Autodesk Inventor part; units mm, degrees
ref_plane "YZ Plane" through (0, 0, 0) normal (1, 0, 0) x (0, 1, 0)
ref_plane "XZ Plane" through (0, 0, 0) normal (0, 1, 0) x (-1, 0, 0)
ref_plane "XY Plane" through (0, 0, 0) normal (0, 0, 1) x (1, 0, 0)
sketch "Sketch1" plane through (0, 0, 0) normal (1, 0, 0) x (0, 1, 0)
  line L0 (44.45, 19.05) -> (-44.45, 19.05)
  line L1 (-44.45, 19.05) -> (-44.45, -19.05)
  line L2 (-44.45, -19.05) -> (44.45, -19.05)
  line L3 (44.45, -19.05) -> (44.45, 19.05)
  line L4 (44.45, 19.05) -> (-44.45, -19.05) construction
  line L5 (-44.45, 19.05) -> (44.45, -19.05) construction
  point P0 (0, 0)
  dimension "d0" = 88.9
  dimension "d1" = 38.1
extrude "Extrusion1" add sketch "Sketch1" along normal mid plane 410
sketch "Sketch2" plane through (-205, -44.45, 19.05) normal (0, 0, 1) x (1, 0, 0)
  line L0 (0, 88.9) -> (0, 0)
  line L1 (0, 67.1803) -> (192.497, 67.1803)
  line L2 (0, 88.9) -> (410, 88.9)
  line L3 (192.497, 88.9) -> (192.497, 67.1803)
  line L4 (192.497, 67.1803) -> (217.497, 67.1803)
  line L5 (217.497, 67.1803) -> (217.497, 88.9)
  point P0 (205, 44.45)
  dimension "d14" = 192.497
  dimension "d15" = 25
extrude "Extrusion2" cut sketch "Sketch2" against normal blind 166.2125 contours L2 L5 L4 L3
properties part number "CNC_1.1v_X_1(faceplate)"
Work out the finished part from the listing and answer in its coordinate system (mm). A direction names the side the tool comes from. Give positions to 0.01 mm unless a question says otherwise; leave off trailing zeros. Loops run counter-clockwise (first coordinate to the right, second up) from the corner with the lowest first, then second, coordinate; pieces in that order, holes last. Notation, with made-up numbers: (-34, -3) - (23, -3) arc R23 ccw to (23, 27) - close; hole circle Ø7 at (71.5, 17.5). An arc over 180 degrees is marked (long way). Answer in a Markdown table with one row per item.
(1) For a pull along X with two mould halves and no side action, classify faces 3 (the face through (205, -1, 0)), 4 (the face through (0, 22.73, 0)), 5 (the face through (-3, -1, -19.05)) as pulls with the +X half, pulls with the -X half, needs draft (parallel to the pull), parting line crosses it, or undercut.
Results list:
| item | result |
|---|---|
| face 3 | pulls with the +X half |
| face 4 | undercut |
| face 5 | needs draft |
(2) Section A-A (y = 36.5) is taken. Give the vertices of the cut face in (x, z).
Results list:
| item | result |
|---|---|
| outline | (-205, -19.05) - (-12.5, -19.05) - (-12.5, 19.05) - (-205, 19.05) - close; (12.5, -19.05) - (205, -19.05) - (205, 19.05) - (12.5, 19.05) - close |
(3) A tool of negligible diameter and unlimited length cuts with its end or side. For faces 1 (the face through (-3, -44.45, 0)), 2 (the face through (-12.503, 34, 0)), from which of +Z, -Z, +X, -X, +Y, -Y can it reach the whole face along a straight path? Write none if from no direction.
Results list:
| item | result |
|---|---|
| face 1 | +Z, -Z, +X, -X, -Y |
| face 2 | +Z, -Z, +Y |
(4) A flat-ended cylindrical pin translates along its axis: pin 1 Ø7.5 at (x, z) = (5.5, -7.5) entering from +Y. Find the tip coordinate at first contact, or state that the pin passes through.
Results list:
| item | result |
|---|---|
| pin 1 | stops at y = 22.73 |
(5) Consider L1, parallel to X at y = 24.5, z = -16.5. Determine where the line is inside the solid, lowest interval first. Write a range as [from, to].
Results list:
| item | result |
|---|---|
| L1 | x = [-205, -12.5], [12.5, 205] |
